from build123d import *

# Parameters (mm, degrees)
BOSS_EXTRUDE1_DEPTH = 5
SKETCH7_R           = 1.25
CUT_EXTRUDE5_DEPTH  = 5
SKETCH9_R           = 7.5
SKETCH9_R_2         = 2.5
CUT_EXTRUDE11_DEPTH = 5


with BuildPart() as part:
    # Sketch3 → Boss-Extrude1 (new body)
    with BuildSketch(Plane(origin=(0, 0, 0), x_dir=(1, 0, 0), z_dir=(0, 1, 0))):
        with BuildLine():
            Line((-60, 40), (-40, 60))
            ThreePointArc((-40, 60), (0, 42.5), (40, 60))
            Line((40, 60), (60, 40))
            ThreePointArc((60, 40), (42.5, 0), (60, -40))
            Line((60, -40), (40, -60))
            ThreePointArc((40, -60), (0, -42.5), (-40, -60))
            Line((-40, -60), (-60, -40))
            ThreePointArc((-60, -40), (-42.5, 0), (-60, 40))
        make_face()
    extrude(amount=BOSS_EXTRUDE1_DEPTH)

    # Sketch7 → Cut-Extrude5 (cut)
    with BuildSketch(Plane(origin=(0, 5, 0), x_dir=(1, 0, 0), z_dir=(0, 1, 0))):
        with BuildLine():
            Line((-47.878679656, 50.707106781), (-49.292893219, 49.292893219))
            Line((-49.292893219, 49.292893219), (-40.807611845, 40.807611845))
            Line((-40.807611845, 40.807611845), (-39.393398282, 42.221825407))
            ThreePointArc((-39.393398282, 42.221825407), (-39.100505063, 42.928932188), (-39.393398282, 43.636038969))
            Line((-39.393398282, 43.636038969), (-46.464466094, 50.707106781))
            ThreePointArc((-46.464466094, 50.707106781), (-47.171572875, 51), (-47.878679656, 50.707106781))
        make_face()
        with BuildLine():
            Line((-40.807611845, 40.807611845), (-49.292893219, 49.292893219))
            Line((-49.292893219, 49.292893219), (-50.707106781, 47.878679656))
            ThreePointArc((-50.707106781, 47.878679656), (-51, 47.171572875), (-50.707106781, 46.464466094))
            Line((-50.707106781, 46.464466094), (-43.636038969, 39.393398282))
            ThreePointArc((-43.636038969, 39.393398282), (-42.928932188, 39.100505063), (-42.221825407, 39.393398282))
            Line((-42.221825407, 39.393398282), (-40.807611845, 40.807611845))
        make_face()
        with Locations(Location((-53.181980515, 41.868272016, 0), (0, 0, 270))):
            Circle(SKETCH7_R)
        with Locations(Location((-48.232233047, 36.918524548, 0), (0, 0, 270))):
            Circle(SKETCH7_R)
        with Locations(Location((-41.868272016, 53.181980515, 0), (0, 0, 270))):
            Circle(SKETCH7_R)
        with Locations(Location((-36.918524548, 48.232233047, 0), (0, 0, 270))):
            Circle(SKETCH7_R)
        with BuildLine():
            Line((-39.393398282, -42.221825407), (-40.807611845, -40.807611845))
            Line((-40.807611845, -40.807611845), (-49.292893219, -49.292893219))
            Line((-49.292893219, -49.292893219), (-47.878679656, -50.707106781))
            ThreePointArc((-47.878679656, -50.707106781), (-47.171572875, -51), (-46.464466094, -50.707106781))
            Line((-46.464466094, -50.707106781), (-39.393398282, -43.636038969))
            ThreePointArc((-39.393398282, -43.636038969), (-39.100505063, -42.928932188), (-39.393398282, -42.221825407))
        make_face()
        with BuildLine():
            Line((-49.292893219, -49.292893219), (-40.807611845, -40.807611845))
            Line((-40.807611845, -40.807611845), (-42.221825407, -39.393398282))
            ThreePointArc((-42.221825407, -39.393398282), (-42.928932188, -39.100505063), (-43.636038969, -39.393398282))
            Line((-43.636038969, -39.393398282), (-50.707106781, -46.464466094))
            ThreePointArc((-50.707106781, -46.464466094), (-51, -47.171572875), (-50.707106781, -47.878679656))
            Line((-50.707106781, -47.878679656), (-49.292893219, -49.292893219))
        make_face()
        with Locations(Location((-53.181980515, -41.868272016, 0), (0, 0, 270))):
            Circle(SKETCH7_R)
        with Locations(Location((-48.232233047, -36.918524548, 0), (0, 0, 270))):
            Circle(SKETCH7_R)
        with Locations(Location((-41.868272016, -53.181980515, 0), (0, 0, 270))):
            Circle(SKETCH7_R)
        with BuildLine():
            Line((49.292893219, -49.292893219), (40.807611845, -40.807611845))
            Line((40.807611845, -40.807611845), (39.393398282, -42.221825407))
            ThreePointArc((39.393398282, -42.221825407), (39.100505063, -42.928932188), (39.393398282, -43.636038969))
            Line((39.393398282, -43.636038969), (46.464466094, -50.707106781))
            ThreePointArc((46.464466094, -50.707106781), (47.171572875, -51), (47.878679656, -50.707106781))
            Line((47.878679656, -50.707106781), (49.292893219, -49.292893219))
        make_face()
        with BuildLine():
            Line((42.221825407, -39.393398282), (40.807611845, -40.807611845))
            Line((40.807611845, -40.807611845), (49.292893219, -49.292893219))
            Line((49.292893219, -49.292893219), (50.707106781, -47.878679656))
            ThreePointArc((50.707106781, -47.878679656), (51, -47.171572875), (50.707106781, -46.464466094))
            Line((50.707106781, -46.464466094), (43.636038969, -39.393398282))
            ThreePointArc((43.636038969, -39.393398282), (42.928932188, -39.100505063), (42.221825407, -39.393398282))
        make_face()
        with Locations(Location((53.181980515, -41.868272016, 0), (0, 0, 270))):
            Circle(SKETCH7_R)
        with BuildLine():
            Line((39.393398282, 42.221825407), (40.807611845, 40.807611845))
            Line((40.807611845, 40.807611845), (49.292893219, 49.292893219))
            Line((49.292893219, 49.292893219), (47.878679656, 50.707106781))
            ThreePointArc((47.878679656, 50.707106781), (47.171572875, 51), (46.464466094, 50.707106781))
            Line((46.464466094, 50.707106781), (39.393398282, 43.636038969))
            ThreePointArc((39.393398282, 43.636038969), (39.100505063, 42.928932188), (39.393398282, 42.221825407))
        make_face()
        with BuildLine():
            Line((49.292893219, 49.292893219), (40.807611845, 40.807611845))
            Line((40.807611845, 40.807611845), (42.221825407, 39.393398282))
            ThreePointArc((42.221825407, 39.393398282), (42.928932188, 39.100505063), (43.636038969, 39.393398282))
            Line((43.636038969, 39.393398282), (50.707106781, 46.464466094))
            ThreePointArc((50.707106781, 46.464466094), (51, 47.171572875), (50.707106781, 47.878679656))
            Line((50.707106781, 47.878679656), (49.292893219, 49.292893219))
        make_face()
        with Locations(Location((41.868272016, 53.181980515, 0), (0, 0, 270))):
            Circle(SKETCH7_R)
        with Locations(Location((36.918524548, 48.232233047, 0), (0, 0, 270))):
            Circle(SKETCH7_R)
        with Locations(Location((53.181980515, 41.868272016, 0), (0, 0, 270))):
            Circle(SKETCH7_R)
        with Locations(Location((48.232233047, 36.918524548, 0), (0, 0, 270))):
            Circle(SKETCH7_R)
        with Locations(Location((-36.918524548, -48.232233047, 0), (0, 0, 90))):
            Circle(SKETCH7_R)
        with Locations(Location((48.232233047, -36.918524548, 0), (0, 0, 90))):
            Circle(SKETCH7_R)
        with Locations(Location((41.868272016, -53.181980515, 0), (0, 0, 270))):
            Circle(SKETCH7_R)
        with Locations(Location((36.918524548, -48.232233047, 0), (0, 0, 270))):
            Circle(SKETCH7_R)
    extrude(amount=-CUT_EXTRUDE5_DEPTH, mode=Mode.SUBTRACT)

    # Sketch9 → Cut-Extrude11 (cut)
    with BuildSketch(Plane(origin=(0, 5, 0), x_dir=(1, 0, 0), z_dir=(0, 1, 0))):
        with Locations(Location((0, 0, 0), (0, 0, 270))):
            Circle(SKETCH9_R)
        with Locations(Location((26.870057685, 26.870057685, 0), (0, 0, 270))):
            Circle(SKETCH9_R_2)
        with Locations(Location((38, 0, 0), (0, 0, 270))):
            Circle(SKETCH9_R_2)
        with Locations(Location((26.870057685, -26.870057685, 0), (0, 0, 270))):
            Circle(SKETCH9_R_2)
        with Locations(Location((0, -38, 0), (0, 0, 270))):
            Circle(SKETCH9_R_2)
        with Locations(Location((-26.870057685, -26.870057685, 0), (0, 0, 270))):
            Circle(SKETCH9_R_2)
        with Locations(Location((-38, 0, 0), (0, 0, 270))):
            Circle(SKETCH9_R_2)
        with Locations(Location((-26.870057685, 26.870057685, 0), (0, 0, 270))):
            Circle(SKETCH9_R_2)
        with Locations(Location((0, 38, 0), (0, 0, 270))):
            Circle(SKETCH9_R_2)
        with Locations(Location((14.142135624, 14.142135624, 0), (0, 0, 270))):
            Circle(SKETCH9_R_2)
        with Locations(Location((19.318516526, -5.176380902, 0), (0, 0, 270))):
            Circle(SKETCH9_R_2)
        with Locations(Location((5.176380902, -19.318516526, 0), (0, 0, 270))):
            Circle(SKETCH9_R_2)
        with Locations(Location((-14.142135624, -14.142135624, 0), (0, 0, 270))):
            Circle(SKETCH9_R_2)
        with Locations(Location((-19.318516526, 5.176380902, 0), (0, 0, 270))):
            Circle(SKETCH9_R_2)
        with Locations(Location((-5.176380902, 19.318516526, 0), (0, 0, 270))):
            Circle(SKETCH9_R_2)
    extrude(amount=-CUT_EXTRUDE11_DEPTH, mode=Mode.SUBTRACT)


solid = part.part
Can you work these out from the model? Positions are in its coordinate system, mm. A direction names the side the tool comes from. Give positions to 0.01 mm unless a question says otherwise; leave off trailing zeros. Order: outer loops, then holes, each group sorted by start corner. A loop starts at its lowest first (then second) coordinate and runs counter-clockwise, first axis right, second up. Notation, with made-up numbers: M 53.25,78.25 L 109.25,78.25 A23 cw 109.25,97.25 Z; hole C -6.5,50.25 d2. An arc over 180 degrees is marked long. Use a Markdown table: item, result. Add a question column.
Item 1: Suppose I cut it at C-C (y = 2.95). Count the separate pieces of the cut face and the enclosed holes in it, then the cut area to 3 significant figures.
Item 2: Will these pins go through, and if not, where does the flat tip stop? pin 1 (12 mm diameter, centred on x = -18.5, z = -14.5, fed in from -Y); pin 2 (2 mm diameter, centred on y = 3, z = 23.5, fed in from +X); pin 3 (2 mm diameter, centred on x = -41.5, y = 0.5, fed in from -Z); pin 4 (1.5 mm diameter, centred on y = 2, z = -23.5, fed in from +X).
Item 3: Suppose I cut it at B-B (x = 0). List the corners of the cut face in (y, z) for me.
Item 4: Suppose I cut it at D-D (x = -32.5). List the corners of the cut face in (y, z) for me, then the cut area to 3 significant figures.
Item 5: We'd pull the mould along Z, two halves only. Please class faces 3 (the cylindrical face through (0.629, 2.465, 42.504)), 4 (the flat face through (14, 0, -1)), 5 (the cylindrical face through (0.33, 2.535, -7.493)): +Z half, -Z half, draft (parallel to the pull), parting line (faces both ways), or undercut.
Item 6: Suppose I cut it at A-A (z = 0). List the corners of the cut face in (x, y) for me.
Item 7: For faces 1 (the flat face through (-50, 2, -50)), 2 (the flat face through (-47.22, 2.54, -42.98)), which set-ups out of +Z, -Z, +X, -X, +Y, -Y let a thin tool reach every point of the face, with its end or its side?
Item 8: If I drill on L1, parallel to Z at x = 29, y = 0.4; L2, parallel to Z at x = 28.5, y = 1; L3, parallel to X at y = 3.05, z = -6, over which ranges is the centre line in solid material (lowest first)? Write a range as [from, to].
Answer sheet:
| question | item | result |
|---|---|---|
| 1 | separate pieces | 1 |
| 1 | enclosed holes | 35 |
| 1 | area | 8,910 mm² |
| 2 | pin 1 | stops at y = 0 |
| 2 | pin 2 | stops at x = 48.32 |
| 2 | pin 3 | stops at z = -59.5 |
| 2 | pin 4 | stops at x = 48.2 |
| 3 | outline | M 0,-42.5 L 5,-42.5 L 5,-40.5 L 0,-40.5 Z; M 0,-35.5 L 5,-35.5 L 5,-7.5 L 0,-7.5 Z; M 0,7.5 L 5,7.5 L 5,35.5 L 0,35.5 Z; M 0,40.5 L 5,40.5 L 5,42.5 L 0,42.5 Z |
| 4 | outline | M 0,-53.26 L 5,-53.26 L 5,53.26 L 0,53.26 Z |
| 4 | area | 533 mm² |
| 5 | face 3 | +Z half |
| 5 | face 4 | draft |
| 5 | face 5 | undercut |
| 6 | outline | M -42.5,0 L -40.5,0 L -40.5,5 L -42.5,5 Z; M -35.5,0 L -7.5,0 L -7.5,5 L -35.5,5 Z; M 7.5,0 L 35.5,0 L 35.5,5 L 7.5,5 Z; M 40.5,0 L 42.5,0 L 42.5,5 L 40.5,5 Z |
| 7 | face 1 | -Z, -X, +Y, -Y |
| 7 | face 2 | +Y, -Y |
| 8 | L1 | z = [-50.86, -28.18], [-25.56, 25.56], [28.18, 50.86] |
| 8 | L2 | z = [-50.55, -28.77], [-24.97, 24.97], [28.77, 50.55] |
| 8 | L3 | x = [-42.83, -21.68], [-16.96, -4.5], [4.5, 42.83] |
